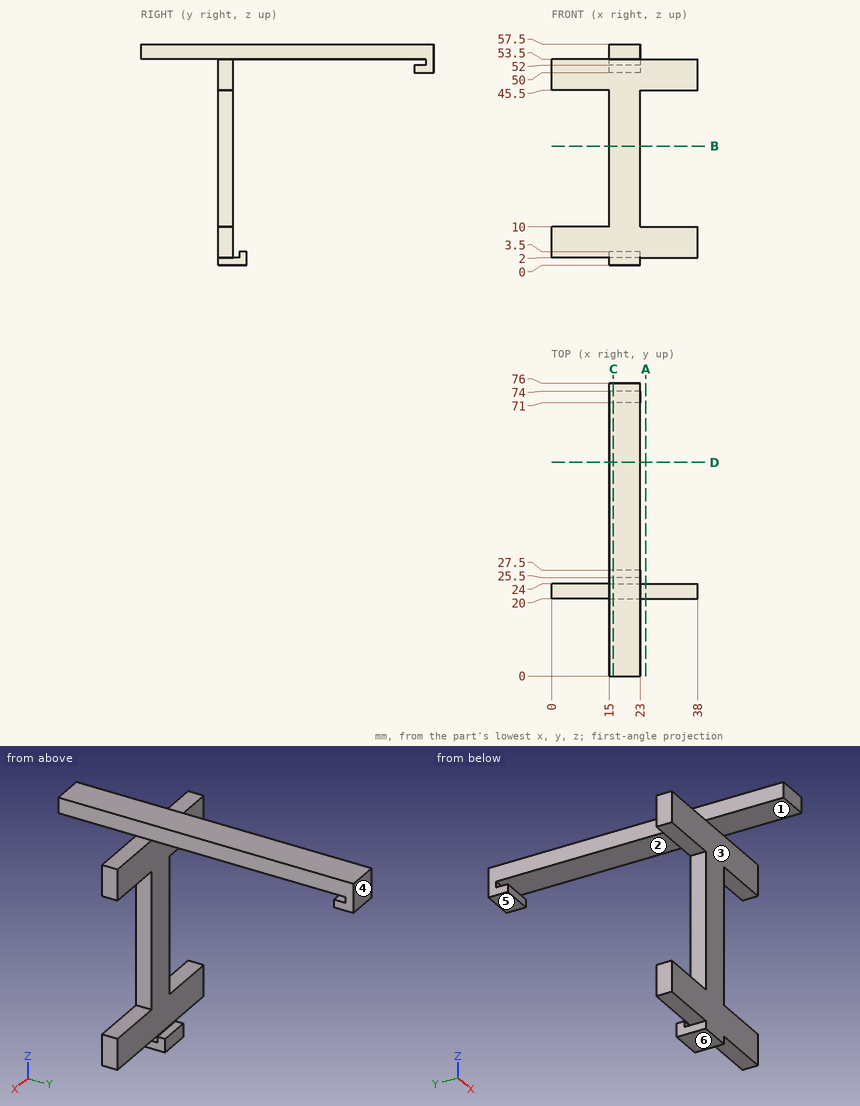
Source: three-view drawing plus pictorial views. Frame: mm from the lowest corner of the part. A direction names the side the tool comes from. Round coordinates to 2 decimals unless told otherwise and drop trailing zeros. Loops run counter-clockwise (first coordinate to the right, second up) from the corner with the lowest first, then second, coordinate; pieces in that order, holes last.
Q1. Mould query, pull axis Y, two halves, no side actions, for the marked faces 1, 2, 3 and 4. Classes: pulls with the +Y half, pulls with the -Y half, needs draft (parallel to the pull), parting line crosses it, or undercut.
Q2. Access query for the marked faces 5 and 6. Directions: +Z, -Z, +X, -X, +Y, -Y. A direction counts if a zero-diameter tool reaches every point of the face in a straight line with its end or side. Return the directions, or none.
Q3. Section A-A, the plane x = 24.5. Return loops of the section in (y, z), plus the area to 3 significant figures.
Q4. Section D-D, the plane y = 55.5. Return loops of the section in (x, z), plus the area to 3 significant figures.
Q5. Section C-C, the plane x = 16. Return loops of the section in (y, z).
Q6. Section B-B, the plane z = 31. Return loops of the section in (x, y).
Q7. First-contact query: P1, Ø4, axis at x = 19.5, z = 1.5, coming from the +Y side; P2, Ø6, axis at x = 23, z = 15, coming from the -Y side; P3, Ø2, axis at y = 22.5, z = 28.5, coming from the -X side. Flat tips, straight axial feed; report the tip coordinate or a pass-through.
Q8. Ray query, line 1 (Z direction, x = 26, y = 23); line 2 (Y direction, x = 19, z = 46); line 3 (Z direction, x = 15.5, y = 48.5). Return the intervals inside material, ascending.
Solutions:
1. face 1: needs draft
1. face 2: undercut
1. face 3: pulls with the -Y half
1. face 4: pulls with the +Y half
2. face 5: -Z, +X, -X, +Y
2. face 6: -Z, +X, -X, +Y, -Y
3. outline: (20, 2) - (24, 2) - (24, 10) - (20, 10) - close; (20, 45.5) - (24, 45.5) - (24, 53.5) - (20, 53.5) - close
3. area: 64.0 mm2
4. outline: (15, 53.5) - (23, 53.5) - (23, 57.5) - (15, 57.5) - close
4. area: 32.0 mm2
5. outline: (0, 53.5) - (20, 53.5) - (20, 0) - (27.5, 0) - (27.5, 3.5) - (25.5, 3.5) - (25.5, 2) - (24, 2) - (24, 53.5) - (74, 53.5) - (74, 52) - (71, 52) - (71, 50) - (76, 50) - (76, 57.5) - (0, 57.5) - close
6. outline: (15, 20) - (23, 20) - (23, 24) - (15, 24) - close
7. P1: stops at y = 27.5
7. P2: stops at y = 20
7. P3: stops at x = 15
8. line 1: z = 2 to 10, 45.5 to 53.5
8. line 2: y = 20 to 24
8. line 3: z = 53.5 to 57.5
